For this review, take the finished solid that the model builds, in its own axes (mm). Face numbers are marked on the shaded views. A direction names the side the tool comes from. Round coordinates to 2 decimals unless told otherwise and drop trailing zeros. Order: outer loops, then holes, each group sorted by start corner. A loop starts at its lowest first (then second) coordinate and runs counter-clockwise, first axis right, second up.
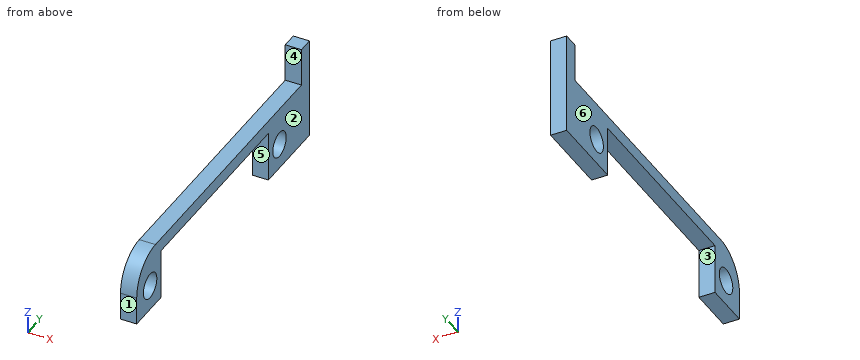
```python
from build123d import *

# Parameters (mm, degrees)
F0_R     = 2.5
F1_DEPTH = 3.175
F2_R     = 7


# Not quite as in the source:
# - a length typed as a fraction of an inch, garbled in the dataset ("3 / 203.2 mm" for 3/8 in), is restored


with BuildPart() as f1:
    # F0 (on Right) → F1 (new body)
    with BuildSketch(Plane.YZ):
        Polygon((-9.125, 0), (0, 0), (0, 9.91), (20, 9.91), (40, 9.91), (40, 0), (52.3, 0), (55.3, 0), (55.3, 20), (52.3, 20), (52.3, 12.5), (-9.125, 12.5), align=None)
        with Locations((-4.125, 5)):
            Circle(F0_R, mode=Mode.SUBTRACT)
        with Locations((44.125, 5)):
            Circle(F0_R, mode=Mode.SUBTRACT)
    extrude(amount=F1_DEPTH)

    # F2
    f2_edges = [f1.edges().sort_by_distance(p)[0] for p in [
        (1.5875, -9.125, 12.5),
    ]]
    fillet(f2_edges, radius=F2_R)


solid = f1.part
```
Q1. Take a section at C-C, the plane z = 6.25. State the section outline as (x, y) points (3 decimals), plus the area to 3 significant figures.
Q2. Mouldability with a two-part tool opening along Y and no side actions: class the marked faces 1, 2 and 3 as +Y half, -Y half, draft (parallel to the pull), parting line (faces both ways), or undercut.
Q3. Tool access review of the marked faces 4, 5 and 6: name each direction out of +Z, -Z, +X, -X, +Y, -Y from which nothing blocks a thin tool from reaching the whole face with its end or side.
Q4. Clearance check with flat-ended pins moving along their axes: pin 1 (4 mm diameter, centred on y = 44.125, z = 5, fed in from +X); pin 2 (8 mm diameter, centred on y = 29, z = 11, fed in from -X); pin 3 (1.6 mm diameter, centred on x = 1.5, z = 17.5, fed in from -Y). State where each tip first meets the part, or that it passes through.
Q5. Take a section at B-B, the plane y = 45. State the section outline as (x, z) points (3 decimals), plus the area to 3 significant figures.
Q6. Take a section at D-D, the plane z = 17.5. State the section outline as (x, y) points (3 decimals), plus the area to 4 significant figures.
Q7. Take a section at A-A, the plane x = 1.9. State the section outline as (y, z) points (3 decimals), plus the area to 3 significant figures.
Q8. Wall thickness on line 1 (Y direction, x = 1.65, z = 1.25) (3 decimals); line 2 (Y direction, x = 0.8, z = 3.25) (3 decimals); line 3 (Z direction, x = 2.1, y = 44): over which ranges is each line inside the solid? List them lowest first.
Working result:
1. outline: (0, -9.085) - (3.175, -9.085) - (3.175, -6.29) - (0, -6.29) - close; (0, -1.96) - (3.175, -1.96) - (3.175, 0) - (0, 0) - close; (0, 40) - (3.175, 40) - (3.175, 41.96) - (0, 41.96) - close; (0, 46.29) - (3.175, 46.29) - (3.175, 55.3) - (0, 55.3) - close
1. area: 49.9 mm2
2. face 1: -Y half
2. face 2: draft
2. face 3: undercut
3. face 4: +Z, +X, -X, -Y
3. face 5: -Z, +X, -X
3. face 6: +Z, -Z, -X, +Y, -Y
4. pin 1: passes through
4. pin 2: stops at x = 0
4. pin 3: stops at y = 52.3
5. outline: (0, 0) - (3.175, 0) - (3.175, 2.658) - (0, 2.658) - close; (0, 7.342) - (3.175, 7.342) - (3.175, 12.5) - (0, 12.5) - close
5. area: 24.8 mm2
6. outline: (0, 52.3) - (3.175, 52.3) - (3.175, 55.3) - (0, 55.3) - close
6. area: 9.525 mm2
7. outline: (-9.125, 0) - (0, 0) - (0, 9.91) - (40, 9.91) - (40, 0) - (55.3, 0) - (55.3, 20) - (52.3, 20) - (52.3, 12.5) - (-2.125, 12.5) arc R7 ccw to (-9.125, 5.5) - close; hole circle Ø5 at (-4.125, 5); hole circle Ø5 at (44.125, 5)
7. area: 382 mm2
8. line 1: y = -9.125 to 0, 40 to 55.3
8. line 2: y = -9.125 to -5.91, -2.34 to 0, 40 to 42.34, 45.91 to 55.3
8. line 3: z = 0 to 2.5, 7.5 to 12.5
